Geometry check sheet. Reference: drawing and pictorial views, mm from the part's lowest x, y, z. Give positions to 0.01 mm unless a question says otherwise; leave off trailing zeros. Loops run counter-clockwise (first coordinate to the right, second up) from the corner with the lowest first, then second, coordinate; pieces in that order, holes last. Notation, with made-up numbers: (-35.75, 71.25) -> (-5.75, 71.25) arc R12 ccw to (-5.75, 92.25) -> close; hole circle Ø1 at (84, -30). An arc over 180 degrees is marked (long way). Write each question's results on one line, items separated by ' | '. Start each with the question number.
1. Cross-section at C-C on y = 159. Record the boundary of the cut face in (x, z).
2. Cross-section at A-A on y = 257.81. Record the boundary of the cut face in (x, z).
3. Cross-section at B-B on x = 0.85. Record the boundary of the cut face in (y, z).
4. Gauge pin test, flat ends, axial feed: pin 1 Ø8 at (y, z) = (191.5, 3) entering from -X; pin 2 Ø1.1 at (x, y) = (2.5, 274) entering from +Z; pin 3 Ø1.5 at (x, z) = (3, 5.5) entering from -Y. Record the tip position at first contact, or that the pin passes through.
5. Material ranges on L1, parallel to Z at x = 1.6, y = 257.81; L2, parallel to Y at x = 1.05, z = 8; L3, parallel to Z at x = 1.9, y = 62, recorded low to high. Write a range as from..to.
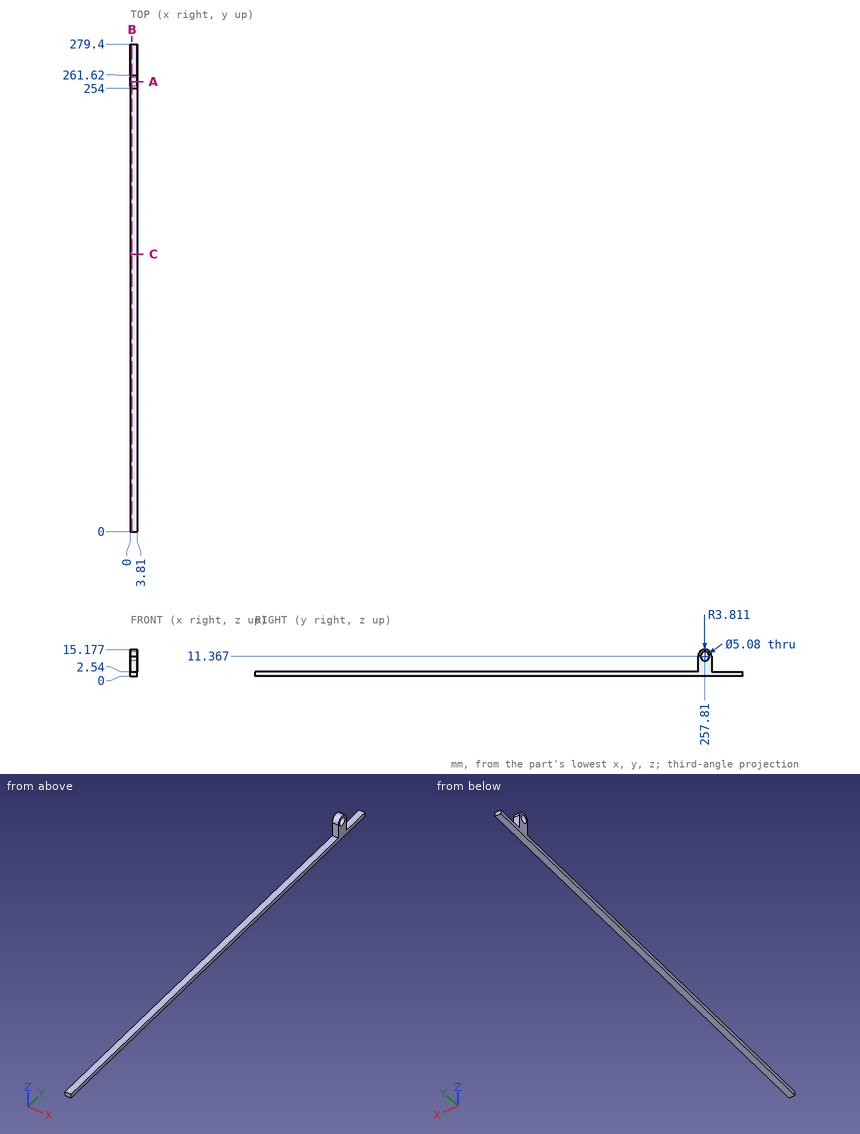
Geometry says:
1) outline: (0, 0) -> (3.81, 0) -> (3.81, 2.54) -> (0, 2.54) -> close
2) outline: (0, 0) -> (3.81, 0) -> (3.81, 8.83) -> (0, 8.83) -> close; (0, 13.91) -> (3.81, 13.91) -> (3.81, 15.18) -> (0, 15.18) -> close
3) outline: (0, 0) -> (279.4, 0) -> (279.4, 2.54) -> (261.62, 2.54) -> (261.62, 11.43) arc R3.81 ccw to (254, 11.43) -> (254, 2.54) -> (0, 2.54) -> close; hole circle Ø5.08 at (257.81, 11.37)
4) pin 1: x = 0 | pin 2: z = 2.54 | pin 3: y = 254
5) L1: 0..8.83, 13.91..15.18 | L2: 254..261.62 | L3: 0..2.54
